Read the model definition and answer for the solid it produces. Units are mm, in the model's axes. Round coordinates to 2 decimals unless told otherwise and drop trailing zeros. Loops run counter-clockwise (first coordinate to the right, second up) from the corner with the lowest first, then second, coordinate; pieces in that order, holes last. Notation, with made-up numbers: M 54,-15.5 L 111,-15.5 A18 cw 111,14.5 Z; hole C 64.25,6.25 d5. An arc over 180 degrees is marked long. Write each question's results on one line, items separated by ' | '.
```python
from build123d import *

# Parameters (mm, degrees)
SKETCH1_R               = 6.35
BOSS_EXTRUDE1_DEPTH     = 25.4
CUT_EXTRUDE2_DEPTH      = 27.940768363
CUT_EXTRUDE2_DEPTH_BACK = 12.7
SKETCH3_R               = 4
SKETCH6_R               = 4.0005
CUT_EXTRUDE5_DEPTH      = 27.940768363
CUT_EXTRUDE3_REACH      = 31.099
CUT_EXTRUDE3_END_RADIUS = 4.0005
SKETCH4_R               = 1.1303


with BuildPart() as part:
    # Sketch1 → Boss-Extrude1 (new body)
    with BuildSketch(Plane(origin=(0, 0, 0), x_dir=(1, 0, 0), z_dir=(0, 1, 0))):
        with Locations(Location((0, 0, 0), (0, 0, 270))):
            Circle(SKETCH1_R)
    extrude(amount=BOSS_EXTRUDE1_DEPTH)

    # Sketch3 → Cut-Extrude2 (cut, two sides: drawn at the far end of the back side and taken through both)
    with BuildSketch(Plane.XZ.offset(-CUT_EXTRUDE2_DEPTH_BACK)):
        with Locations(Location((0, 0, 0), (0, 0, 90))):
            Circle(SKETCH3_R)
    extrude(amount=CUT_EXTRUDE2_DEPTH + CUT_EXTRUDE2_DEPTH_BACK, mode=Mode.SUBTRACT)

    # Sketch6 → Cut-Extrude5 (cut, through all)
    with BuildSketch(Plane(origin=(0, 0, 0), x_dir=(-1, 0, 0), z_dir=(0, -1, 0))):
        with Locations(Location((0, 0, 0), (0, 0, 90))):
            Circle(SKETCH6_R)
    extrude(amount=-CUT_EXTRUDE5_DEPTH, mode=Mode.SUBTRACT)

    # Cut-Extrude3: up to this cylinder (the profile starts outside it)
    cut_extrude3_end = Plane(origin=(0, 12.7, 0), z_dir=(0, -1, 0)) * Cylinder(CUT_EXTRUDE3_END_RADIUS, 83.899, mode=Mode.PRIVATE)
    # Sketch4 → Cut-Extrude3 (cut, up to the surface)
    with BuildSketch(Plane.XY.offset(6.35), mode=Mode.PRIVATE) as cut_extrude3_sk1:
        with Locations((0, 6.35)):
            Circle(SKETCH4_R)
    cut_extrude3_tool1 = extrude(cut_extrude3_sk1.sketch, amount=-CUT_EXTRUDE3_REACH, mode=Mode.PRIVATE) - cut_extrude3_end
    add(cut_extrude3_tool1.solids().sort_by_distance((0, 6.35, 6.35))[0], mode=Mode.SUBTRACT)
    # Sketch4 → Cut-Extrude3 (cut, up to the surface)
    with BuildSketch(Plane.XY.offset(6.35), mode=Mode.PRIVATE) as cut_extrude3_sk2:
        with Locations((0, 19.05)):
            Circle(SKETCH4_R)
    cut_extrude3_tool2 = extrude(cut_extrude3_sk2.sketch, amount=-CUT_EXTRUDE3_REACH, mode=Mode.PRIVATE) - cut_extrude3_end
    add(cut_extrude3_tool2.solids().sort_by_distance((0, 19.05, 6.35))[0], mode=Mode.SUBTRACT)


solid = part.part
```
1. Find the intervals of material crossed by L1, parallel to Y at x = 0, z = 4.5; L2, parallel to X at y = 16, z = -1.75; L3, parallel to X at y = 6, z = 0, in increasing order.
Completed:
L1: y = 0 to 5.22, 7.48 to 17.92, 20.18 to 25.4 | L2: x = -6.1 to -3.6, 3.6 to 6.1 | L3: x = -6.35 to -4, 4 to 6.35
2. Determine the mould class of faces 1 (the face through (0.522, 18.047, 5.111)), 2 (the face through (-4.1, 25.4, 1.3)), 3 (the face through (-0.245, 5.247, 5.111)), 4 (the face through (-4.1, 0, 1.3)) for opening direction Y: released by +Y, released by -Y, zero draft, split by the parting line, or undercut.
Completed:
face 1: undercut | face 2: released by +Y | face 3: undercut | face 4: released by -Y
3. Given P1, Ø1, axis at y = 9, z = -1, coming from the +X side; P2, Ø1.8, axis at x = 0, y = 19.05, coming from the +Z side; P3, Ø1.5, axis at x = -3, y = 22.5, coming from the -Z side, each flat-ended and moving along its own axis, determine where each tip first touches the part or whether it passes through.
Completed:
P1: stops at x = 6.33 | P2: stops at z = -3.9 | P3: stops at z = -5.94
4. Find section A-A, the plane z = 0. Give the vertices of the cut face in (x, y), then the cut area to 3 significant figures.
Completed:
outline: M -6.35,0 L -4,0 L -4,25.4 L -6.35,25.4 Z; M 4,0 L 6.35,0 L 6.35,25.4 L 4,25.4 Z | area: 119 mm2
5. Find section D-D, the plane y = 9.5. Give the vertices of the cut face in (x, z).
Completed:
outline: C 0,0 d12.7; hole C 0,0 d8
6. Find section B-B, the plane x = 0. Give the vertices of the cut face in (y, z).
Completed:
outline: M 0,-6.35 L 25.4,-6.35 L 25.4,-4 L 0,-4 Z; M 0,4 L 5.22,4 L 5.22,6.35 L 0,6.35 Z; M 7.48,4 L 17.92,4 L 17.92,6.35 L 7.48,6.35 Z; M 20.18,4 L 25.4,4 L 25.4,6.35 L 20.18,6.35 Z
7. Find section C-C, the plane x = 2.5. Give the vertices of the cut face in (y, z), then the cut area to 3 significant figures.
Completed:
outline: M 0,-5.84 L 25.4,-5.84 L 25.4,-3.12 L 0,-3.12 Z; M 0,3.12 L 25.4,3.12 L 25.4,5.84 L 0,5.84 Z | area: 138 mm2
